```python
from build123d import *

# Parameters (mm, degrees)
F0_R     = 2.55
F1_DEPTH = 6.35


with BuildPart() as f1:
    # F0 (on Top) → F1 (new body)
    with BuildSketch(Plane.XY):
        with BuildLine():
            Line((-8.919358, 346.191724), (-140.330109, -45.140431))
            ThreePointArc((-140.330109, -45.140431), (-139.649673, -49.651147), (-135.590217, -51.732103))
            Line((-135.590217, -51.732103), (-75.093617, -51.732103))
            Line((-75.093617, -51.732103), (-75.093617, -46.732103))
            Line((-75.093617, -46.732103), (-76.543617, -46.732103))
            Line((-76.543617, -46.732103), (-76.543617, -42.732103))
            Line((-76.543617, -42.732103), (-75.093617, -42.732103))
            Line((-75.093617, -42.732103), (-72.543617, -42.732103))
            Line((-72.543617, -42.732103), (-69.993617, -42.732103))
            Line((-69.993617, -42.732103), (-68.543617, -42.732103))
            Line((-68.543617, -42.732103), (-68.543617, -46.732103))
            Line((-68.543617, -46.732103), (-69.993617, -46.732103))
            Line((-69.993617, -46.732103), (-69.993617, -51.732103))
            Line((-69.993617, -51.732103), (-52.543617, -51.732103))
            Line((-52.543617, -51.732103), (-52.543617, -58.032103))
            Line((-52.543617, -58.032103), (-2.543617, -58.032103))
            Line((-2.543617, -58.032103), (-2.543617, -51.732103))
            Line((-2.543617, -51.732103), (2.456383, -51.732103))
            Line((2.456383, -51.732103), (7.456383, -51.732103))
            Line((7.456383, -51.732103), (7.456383, -58.032103))
            Line((7.456383, -58.032103), (57.456383, -58.032103))
            Line((57.456383, -58.032103), (57.456383, -51.732103))
            Line((57.456383, -51.732103), (74.906383, -51.732103))
            Line((74.906383, -51.732103), (74.906383, -46.732103))
            Line((74.906383, -46.732103), (73.456383, -46.732103))
            Line((73.456383, -46.732103), (73.456383, -42.732103))
            Line((73.456383, -42.732103), (74.906383, -42.732103))
            Line((74.906383, -42.732103), (77.456383, -42.732103))
            Line((77.456383, -42.732103), (80.006383, -42.732103))
            Line((80.006383, -42.732103), (81.456383, -42.732103))
            Line((81.456383, -42.732103), (81.456383, -46.732103))
            Line((81.456383, -46.732103), (80.006383, -46.732103))
            Line((80.006383, -46.732103), (80.006383, -51.732103))
            Line((80.006383, -51.732103), (140.566313, -51.732103))
            ThreePointArc((140.566313, -51.732103), (144.588797, -49.6701), (145.263036, -45.200466))
            Line((145.263036, -45.200466), (13.832124, 346.191724))
            ThreePointArc((13.832124, 346.191724), (2.456383, 354.371709), (-8.919358, 346.191724))
        make_face()
        with BuildLine():
            Line((66.796947, -1.732103), (2.456383, -1.732103))
            Line((2.456383, -1.732103), (-61.88418, -1.732103))
            ThreePointArc((-61.88418, -1.732103), (-68.37931, 1.597426), (-69.468008, 8.814573))
            Line((-69.468008, 8.814573), (-5.127444, 200.416334))
            ThreePointArc((-5.127444, 200.416334), (2.456383, 205.869657), (10.040211, 200.416334))
            Line((10.040211, 200.416334), (74.380774, 8.814573))
            ThreePointArc((74.380774, 8.814573), (73.292076, 1.597426), (66.796947, -1.732103))
        make_face(mode=Mode.SUBTRACT)
        with Locations((2.456383, 329.067897)):
            Circle(F0_R, mode=Mode.SUBTRACT)
    extrude(amount=F1_DEPTH)


solid = f1.part
```
Design review of the part built by this model. Coordinates are the model's own, in mm. A direction names the side the tool comes from. Coordinates: 2 decimals unless noted, no trailing zeros. Write each loop counter-clockwise with the first axis right and the second up, starting at its lowest first coordinate (ties: lowest second). Pieces come first, ordered by that corner, then holes. Notation, with made-up numbers: M 0,29 L 5,29 A22 ccw 5,64 Z; hole C 58.25,45.5 d11. An arc over 180 degrees is marked long. Answer as a JSON object with one key per item and string values.
Item 1: Add section B-B, the plane y = 96. Give the boundary of the cut face in (x, z), and give its area (3 significant figures).
Outcome:
{"outline": "M -92.93,0 L -40.19,0 L -40.19,6.35 L -92.93,6.35 Z; M 45.1,0 L 97.85,0 L 97.85,6.35 L 45.1,6.35 Z", "area": "670 mm²"}
Item 2: Wall thickness on probe 1 along Y at (x, z) = (1.5, 2.75); probe 2 along X at (y, z) = (19, 3.5); probe 3 along X at (y, z) = (202, 5.25): over which ranges is each line inside the solid? List them lowest first.
Outcome:
{"probe 1": "-51.73 to -1.73, 205.81 to 326.7, 331.43 to 354.33", "probe 2": "-118.79 to -66.05, 70.96 to 123.7", "probe 3": "-57.34 to -4.39, 9.31 to 62.25"}
Item 3: Add section C-C, the plane z = 3.5. State how many separate pieces and enclosed holes the cut face has, and give its area (3 significant figures).
Outcome:
{"separate pieces": "1", "enclosed holes": "2", "area": "46,000 mm²"}
Item 4: Add section D-D, the plane y = 282. Give the boundary of the cut face in (x, z).
Outcome:
{"outline": "M -30.48,0 L 35.39,0 L 35.39,6.35 L -30.48,6.35 Z"}
Item 5: Add section A-A, the plane x = 26. Give the boundary of the cut face in (y, z).
Outcome:
{"outline": "M -58.03,0 L -1.73,0 L -1.73,6.35 L -58.03,6.35 Z; M 152.89,0 L 309.96,0 L 309.96,6.35 L 152.89,6.35 Z"}
Item 6: Insertion check: pin 1 Ø3 at (y, z) = (-54.5, 4) entering from +X; pin 2 Ø3 at (y, z) = (-45, 2) entering from -X; pin 3 Ø1 at (y, z) = (83, 1) entering from +X. Each pin has a flat end and moves straight along its axis. Give the tip position at first contact, or say it passes through.
Outcome:
{"pin 1": "x = 57.46", "pin 2": "x = -140.58", "pin 3": "x = 102.38"}
Item 7: Machinability: for faces 1 (the flat face through (-37.75, 103.27, 3.13)), 2 (the flat face through (-51, 103, 6.35)), which of the approach directions +Z, -Z, +X, -X, +Y, -Y give a long, thin tool a straight path to every point of the face, cutting with its end or side? Answer none if there is none.
Outcome:
{"face 1": "+Z, -Z", "face 2": "+Z, +X, -X, +Y, -Y"}
Item 8: Draft analysis for pull direction Y (two halves, no side actions). For faces 3 (the flat face through (-51, 103, 0)), 4 (the flat face through (80.468, 147.756, 3.131)), 5 (the cylindrical face through (-68.317, 1.512, 3.131)), state which applies: pulls with the +Y half, pulls with the -Y half, needs draft (parallel to the pull), parting line crosses it, or undercut.
Outcome:
{"face 3": "needs draft", "face 4": "pulls with the +Y half", "face 5": "undercut"}
